Here's the drawing with two shaded views (mm, measured from the low corner). I have some questions. Give positions to 0.01 mm unless a question says otherwise; leave off trailing zeros. Write each loop counter-clockwise with the first axis right and the second up, starting at its lowest first coordinate (ties: lowest second). Pieces come first, ordered by that corner, then holes.
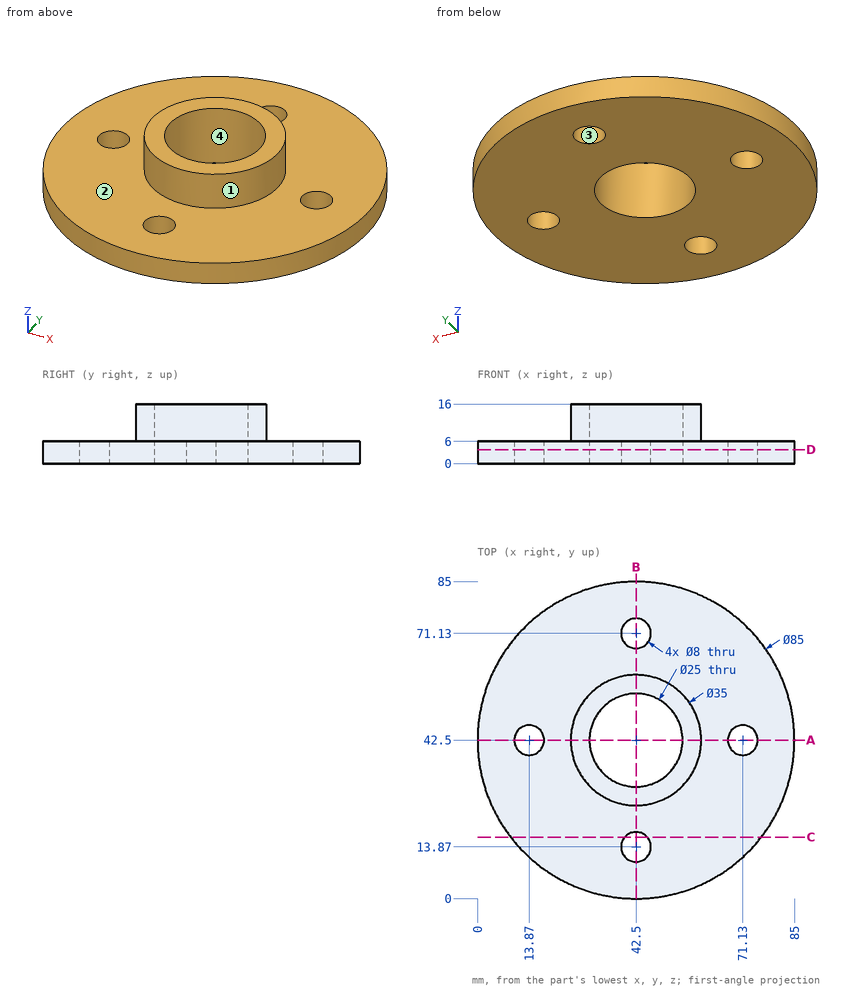
(1) Imagine slicing it at A-A, the plane y = 42.5. Write out the boundary of the cut face in (x, z), plus the area to 3 significant figures.
Returned:
outline: (0, 0) - (9.87, 0) - (9.87, 6) - (0, 6) - close; (17.87, 0) - (30, 0) - (30, 16) - (25, 16) - (25, 6) - (17.87, 6) - close; (55, 0) - (67.13, 0) - (67.13, 6) - (60, 6) - (60, 16) - (55, 16) - close; (75.13, 0) - (85, 0) - (85, 6) - (75.13, 6) - close
area: 364 mm2
(2) If we mould it in two halves opening along Y, with no side actions, what happens to the marked faces 1, 2, 3 and 4? For each: +Y half, -Y half, draft (parallel to the pull), parting line (faces both ways), or undercut.
Returned:
face 1: parting line
face 2: draft
face 3: undercut
face 4: undercut
(3) Imagine slicing it at D-D, the plane z = 3.75. Write out the boundary of the cut face in (x, y).
Returned:
outline: circle Ø85 at (42.5, 42.5); hole circle Ø8 at (13.87, 42.5); hole circle Ø25 at (42.5, 42.5); hole circle Ø8 at (42.5, 13.87); hole circle Ø8 at (42.5, 71.13); hole circle Ø8 at (71.13, 42.5)
(4) If I drill on L1, parallel to Y at x = 42.5, z = 11.25; L2, parallel to Z at x = 17, y = 30; L3, parallel to Y at x = 48.5, z = 15 (1 decimal), over which ranges is the centre line in solid material (lowest first)?
Returned:
L1: y = 25 to 30, 55 to 60
L2: z = 0 to 6
L3: y = 26.1 to 31.5, 53.5 to 58.9
(5) Imagine slicing it at C-C, the plane y = 16.5. Write out the boundary of the cut face in (x, z).
Returned:
outline: (8.88, 0) - (39.49, 0) - (39.49, 6) - (8.88, 6) - close; (45.51, 0) - (76.12, 0) - (76.12, 6) - (45.51, 6) - close
(6) Will these pins go through, and if not, where does the flat tip stop? P1, Ø7, axis at x = 13.87, y = 42.5, coming from the +Z side; P2, Ø9, axis at x = 71.13, y = 42.5, coming from the +Z side; P3, Ø6, axis at x = 62.5, z = 6.5, coming from the +Y side; P4, Ø8, axis at y = 68.5, z = 3.5, coming from the +X side.
Returned:
P1: passes through
P2: stops at z = 6
P3: stops at y = 81.43
P4: stops at x = 78.86
